Can you work these out from the model? Positions are in its coordinate system, mm. A direction names the side the tool comes from. Give positions to 0.01 mm unless a question says otherwise; leave off trailing zeros. Order: outer loops, then holes, each group sorted by start corner. A loop starts at its lowest first (then second) coordinate and runs counter-clockwise, first axis right, second up. Notation, with made-up numbers: (66, -19) - (119, -19) arc R23 ccw to (119, -5) - close; hole circle Ø5 at (65, -25.5). An arc over 180 degrees is marked (long way). Return JSON: item names as keys, results as strings.
Autodesk Inventor part; units mm, degrees
ref_plane "YZ Plane" through (0, 0, 0) normal (1, 0, 0) x (0, 1, 0)
ref_plane "XZ Plane" through (0, 0, 0) normal (0, 1, 0) x (-1, 0, 0)
ref_plane "XY Plane" through (0, 0, 0) normal (0, 0, 1) x (1, 0, 0)
sketch "Sketch1" plane through (0, 0, 0) normal (0, 0, 1) x (1, 0, 0)
  line L0 (0, 0) -> (82.5, 0)
  line L1 (82.5, 0) -> (82.5, 58)
  line L2 (82.5, 58) -> (0, 58)
  line L3 (0, 58) -> (0, 0)
  line L4 (12.6, 10) -> (68.5, 10) construction
  line L5 (68.5, 10) -> (68.5, 48) construction
  line L6 (68.5, 48) -> (12.6, 48) construction
  line L7 (12.6, 48) -> (12.6, 10) construction
  circle A0 centre (12.6, 48) radius 2
  circle A1 centre (12.6, 10) radius 2
  circle A2 centre (68.5, 10) radius 2
  circle A3 centre (54.5, 48) radius 2
  circle A4 centre (23.5, 29) radius 12.5
  circle A5 centre (23.5, 29) radius 5
  point P0 (12.6, 29)
  point P1 (0, 29)
  dimension "d0" = 82.5
  dimension "d1" = 58
  dimension "d2" = 38
  dimension "d3" = 55.9
  dimension "d4" = 12.6
  dimension "d5" = 4
  dimension "d6" = 4
  dimension "d7" = 4
  dimension "d8" = 4
  dimension "d9" = 25
  dimension "d10" = 41.9
  dimension "d11" = 10.9
  dimension "d12" = 10
extrude "Extrusion1" add sketch "Sketch1" along normal blind 44 contours L3 L2 L1 L0 | A4 | A5
extrude "Extrusion2" add sketch "Sketch1" along normal blind 49 and the other way blind 5 contours A4
extrude "Extrusion3" add sketch "Sketch1" against normal blind 25 and the other way blind 69 contours A5
sketch "Sketch2" plane through (0, 0, 44) normal (0, 0, 1) x (1, 0, 0)
  circle A0 centre (12.6, 48) radius 2
  circle A1 centre (54.5, 48) radius 2
  circle A2 centre (68.5, 10) radius 2
  circle A3 centre (12.6, 10) radius 2
  circle A4 centre (12.6, 48) radius 5
  circle A5 centre (54.5, 48) radius 5
  circle A6 centre (68.5, 10) radius 5
  circle A7 centre (12.6, 10) radius 5
  point P0 (0, 0)
  dimension "d23" = 10
  dimension "d24" = 10
  dimension "d25" = 10
  dimension "d26" = 10
extrude "Extrusion4" add sketch "Sketch2" along normal blind 2.5
sketch "Sketch3" plane through (0, 0, 0) normal (0, 0, -1) x (-1, 0, 0)
  circle A0 centre (-12.6, 48) radius 2
  circle A1 centre (-12.6, 48) radius 5
  circle A2 centre (-12.6, 10) radius 2
  circle A3 centre (-12.6, 10) radius 5
  circle A4 centre (-54.5, 48) radius 2
  circle A5 centre (-54.5, 48) radius 5
  circle A6 centre (-68.5, 10) radius 2
  circle A7 centre (-68.5, 10) radius 5
  point P0 (0, 0)
extrude "Extrusion5" add sketch "Sketch3" along normal blind 2.5
sketch "Sketch4" plane through (82.5, 0, 0) normal (1, 0, 0) x (0, 0, -1)
  circle A0 centre (-22, 29) radius 22
  line L0 (0, 0) -> (0, 58)
  line L1 (0, 58) -> (-44, 58)
  point P0 (-22, 58)
  point P1 (0, 29)
  dimension "d31" = 44
extrude "Extrusion6" add sketch "Sketch4" along normal blind 66.5
sketch "Sketch5" plane through (23.5, 29, -25) normal (0, 0, -1) x (-1, 0, 0)
  circle A0 centre (0, 0) radius 5
  line L0 (4.25, -2.6339) -> (4.25, 2.6339)
  arc A1 (4.25, -2.6339) -> (4.25, 2.6339) centre (0, 0) ccw
  point P0 (23.5, -29)
  point P1 (4.25, 0)
  dimension "d34" = 4.25
extrude "Extrusion7" cut sketch "Sketch5" against normal blind 15 contours A0 L0 picked at (4.3873, -0.6025)
sketch "Sketch6" plane through (23.5, 29, 69) normal (0, 0, 1) x (1, 0, 0)
  circle A0 centre (0, 0) radius 5
  line L0 (-4.25, 2.6339) -> (-4.25, -2.6339)
  arc A1 (-4.25, 2.6339) -> (-4.25, -2.6339) centre (0, 0) ccw
  point P0 (-23.5, -29)
  point P1 (-4.25, 0)
  dimension "d37" = 4.25
extrude "Extrusion8" cut sketch "Sketch6" against normal blind 15 contours L0 A0 picked at (-4.4085, 0.5446)
fillet "Fillet1" radius 4 4 edges at (82.5, 58, 22) (0, 58, 22) (82.5, 0, 22) (0, 0, 22)
properties part number "TJW83FZY4468-527i" material "Stainless Steel"
1. Suppose I cut it at B-B (z = 22). List the corners of the cut face in (x, y) for me.
Checks:
{"outline": "(0, 4) arc R4 ccw to (4, 0) - (78.5, 0) arc R4 ccw to (82.5, 4) - (82.5, 7) - (149, 7) - (149, 51) - (82.5, 51) - (82.5, 54) arc R4 ccw to (78.5, 58) - (4, 58) arc R4 ccw to (0, 54) - close; hole circle Ø4 at (12.6, 10); hole circle Ø4 at (12.6, 48); hole circle Ø4 at (54.5, 48); hole circle Ø4 at (68.5, 10)"}
2. Suppose I cut it at D-D (y = 18). List the corners of the cut face in (x, z) for me.
Checks:
{"outline": "(0, 0) - (17.56, 0) - (17.56, -5) - (29.44, -5) - (29.44, 0) - (82.5, 0) - (82.5, 2.95) - (149, 2.95) - (149, 41.05) - (82.5, 41.05) - (82.5, 44) - (29.44, 44) - (29.44, 49) - (17.56, 49) - (17.56, 44) - (0, 44) - close"}
3. If I drill on L1, parallel to Y at x = 12.6, z = 31.5; L2, parallel to X at y = 10, z = 33; L3, parallel to X at y = 48, z = 19, over which ranges is the centre line in solid material (lowest first)? Write a range as [from, to].
Checks:
{"L1": "[0, 8], [12, 46], [50, 58]", "L2": "[0, 10.6], [14.6, 66.5], [70.5, 149]", "L3": "[0, 10.6], [14.6, 52.5], [56.5, 149]"}
4. Thinking about a two-plate mould opening in Y: for faces 6 (the face through (1.141, 1.203, 22.308)), 7 (the face through (28.119, 27.085, -14.86)), 8 (the face through (71, 10, 46.5)), 9 (the face through (15.288, 43.784, 45.232)), which applies, +Y half, -Y half, draft (parallel to the pull), parting line (faces both ways), or undercut?
Checks:
{"face 6": "-Y half", "face 7": "parting line", "face 8": "draft", "face 9": "undercut"}
5. For pin 1 Ø5 at (x, y) = (12.6, 10) entering from +Z; pin 2 Ø10 at (x, z) = (101.5, 33.5) entering from -Y; pin 3 Ø12 at (y, z) = (52, 26.5) entering from +X; pin 4 Ø6 at (y, z) = (27.5, 59.5) entering from -X, each with a flat end and sliding along its axis, tell me the tip position at first contact or that it passes through.
Checks:
{"pin 1": "z = 46.5", "pin 2": "y = 7.98", "pin 3": "x = 149", "pin 4": "x = 19.25"}
6. Suppose I cut it at C-C (y = 48). State how many separate pieces and enclosed holes the cut face has, plus the area to 3 significant figures.
Checks:
{"separate pieces": "3", "enclosed holes": "0", "area": "4,810 mm^2"}
7. On a 3-axis mill with a long thin cutter (end or side, diameter ignored), from which of +Z, -Z, +X, -X, +Y, -Y can I reach the whole of each face in a straight line? I mean faces 1 (the face through (13.251, 43.043, -1.232)), 2 (the face through (19.25, 29, -18)), 3 (the face through (10, 10, -2.5)), 4 (the face through (41, 29, 44)), 5 (the face through (82.5, 6, 22)). Say none if no direction works.
Checks:
{"face 1": "-Z", "face 2": "-Z, -X, +Y, -Y", "face 3": "-Z, +X, -X, -Y", "face 4": "+Z", "face 5": "+X, -Y"}
8. Suppose I cut it at A-A (x = 68.5). List the corners of the cut face in (y, z) for me, plus the area to 3 significant figures.
Checks:
{"outline": "(0, 0) - (5, 0) - (5, -2.5) - (8, -2.5) - (8, 46.5) - (5, 46.5) - (5, 44) - (0, 44) - close; (12, -2.5) - (15, -2.5) - (15, 0) - (58, 0) - (58, 44) - (15, 44) - (15, 46.5) - (12, 46.5) - close", "area": "2,410 mm^2"}
